Geometry: final body of the model. Coordinates: model frame, mm. Face numbers are marked on the shaded views. A direction names the side the tool comes from. Coordinates: 2 decimals unless noted, no trailing zeros. Order: outer loops, then holes, each group sorted by start corner. A loop starts at its lowest first (then second) coordinate and runs counter-clockwise, first axis right, second up. Notation, with made-up numbers: M 45.25,78 L 68.25,78 A27 ccw 68.25,98 Z; hole C 1.25,60 d9. An arc over 180 degrees is marked long. One line per question, with ' | ' between items.
Autodesk Inventor part; units mm, degrees
ref_plane "YZ Plane" through (0, 0, 0) normal (1, 0, 0) x (0, 1, 0)
ref_plane "XZ Plane" through (0, 0, 0) normal (0, 1, 0) x (-1, 0, 0)
ref_plane "XY Plane" through (0, 0, 0) normal (0, 0, 1) x (1, 0, 0)
sketch "Sketch1" plane through (0, 0, 0) normal (0, 1, 0) x (-1, 0, 0)
  line L0 (55, 40) -> (-55, 40)
  line L1 (-55, 40) -> (-55, -40)
  line L2 (-55, -40) -> (55, -40)
  line L3 (55, -40) -> (55, 40)
  line L4 (55, 40) -> (-55, -40) construction
  line L5 (-55, 40) -> (55, -40) construction
  line L6 (0, -56) -> (0, 56)
  point P0 (0, 0)
  dimension "d0" = 110
  dimension "d1" = 80
extrude "Extrusion1" add sketch "Sketch1" along normal blind 3
sketch "Sketch2" plane through (0, 3, 0) normal (0, 1, 0) x (1, 0, 0)
  line L0 (-55, 40) -> (-55, -40)
  line L1 (-55, -40) -> (55, -40)
  line L2 (55, -40) -> (55, 40)
  line L3 (49, -34) -> (-49, -34)
  line L4 (-49, -34) -> (-49, 34)
  line L5 (-49, 34) -> (49, 34)
  line L6 (49, 34) -> (49, -34)
  line L7 (49, -34) -> (-49, 34) construction
  line L8 (-49, -34) -> (49, 34) construction
  line L9 (55, 40) -> (-55, 40)
  point P0 (0, 0)
  dimension "d36" = 98
  dimension "d37" = 68
extrude "Extrusion2" add sketch "Sketch2" along normal blind 25.4125
sketch "Sketch7" plane through (-49, 3, 34) normal (1, 0, 0) x (0, 0, -1)
  circle A0 centre (31.25, 12) radius 8.25
  line L0 (74, -3) -> (-6, -3)
  circle A1 centre (31.25, 12) radius 10.25
  line L1 (21, 12) -> (41.5, 12)
  line L2 (41.5, 12) -> (41.5, 0)
  line L3 (-6, -3) -> (-6, 25.4125)
  line L4 (0, 0) -> (41.5, 0)
  line L5 (0, 0) -> (0, 25.4125)
  line L6 (21, 12) -> (21, 0)
  line L7 (68, 0) -> (0, 0)
  point P0 (34, -3)
  point P1 (54, -3)
  point P2 (0, 25.25)
  point P3 (22.1693, 16.7543)
  point P4 (23, 12)
  point P5 (39.5, 12)
  dimension "MotorDiameter" = 16.5
  dimension "d18" = 15
  dimension "d20" = 2
  dimension "d144" = 37.25
extrude "Extrusion5" add sketch "Sketch7" along normal blind 13 contours L1 A1 A0 | A0 L1 A1 | L2 L4 L6 A1
sketch "Sketch8" plane through (-36, 3, 34) normal (1, 0, 0) x (0, 0, -1)
  arc A0 (41.5, 12) -> (21, 12) centre (31.25, 12) ccw
  arc A1 (41.5, 12) -> (21, 12) centre (31.25, 12) ccw
  arc A2 (23, 12) -> (23, 12) centre (31.25, 12) ccw
  line L0 (41.5, 0) -> (21, 0)
  line L1 (21, 12) -> (21, 0)
  line L2 (41.5, 0) -> (21, 0)
  line L3 (41.5, 0) -> (41.5, 12)
  circle A3 centre (31.25, 12) radius 7.75
  line L4 (25.15, 17.5545) -> (25.15, 0)
  line L5 (31.25, 19.75) -> (31.25, 4.25)
  line L6 (37.35, 17.5545) -> (37.35, 0)
  circle A4 centre (31.25, 12) radius 8.25
  arc A5 (41.5, 12) -> (21, 12) centre (31.25, 12) ccw
  line L7 (21, 12) -> (21, 0)
  line L8 (41.5, 0) -> (21, 0)
  line L9 (41.5, 0) -> (41.5, 12)
  line L10 (37.35, 17.5545) -> (39.8645, 17.5545)
  line L11 (25.15, 17.5545) -> (22.6355, 17.5545)
  point P0 (34, -3)
  point P1 (19.75, 15)
  point P2 (37.35, 7.2196)
  point P3 (25.15, 7.2196)
  point P4 (22.6355, 17.5545)
  dimension "d145" = 15.5
  dimension "d146" = 15.5
  dimension "d147" = 12.2
extrude "Extrusion6" add sketch "Sketch8" along normal blind 20 contours L3 L0 L6 A2 L10 A0 | L11 A2 L4 L0 L1 A0 | A2 L6 A3 | L0 L4 A2 L6 | L4 A3 A2 | A3 L6 | A2 L4 A3 L6 | L4 A3 picked at (32.1563, 4.1687)
sketch "Sketch9" plane through (-49, 17, 8.75) normal (1, 0, 0) x (0, 0, -1)
  line L0 (48.75, -17) -> (-31.25, -17)
  line L1 (-31.25, -17) -> (-31.25, 11.4125)
  arc A0 (-0.1, 3.5545) -> (12.1, 3.5545) centre (6, -2) ccw
  arc A1 (12.1, 3.5545) -> (-0.1, 3.5545) centre (6, -2) ccw
  circle A2 centre (6, -2) radius 8.25
  circle A3 centre (6, -2) radius 1.75
  point P0 (8.75, -17)
  point P1 (44, -20)
  dimension "d148" = 3.5
extrude "Extrusion7" cut sketch "Sketch9" against normal up to surface (6 mm away) contours A3
mirror "Mirror2" about plane through (0, 0, 0) normal (1, 0, 0) of "Extrusion7", "Extrusion6", "Extrusion5"
sketch "Sketch28" plane through (-49, 3, -34) normal (0, 0, 1) x (1, 0, 0)
  line L0 (98, 0) -> (0, 0)
  line L1 (98, 0) -> (98, 25.4125)
  line L2 (0, 0) -> (0, 25.4125)
  line L3 (92, 19.4125) -> (92, 6)
  line L4 (92, 6) -> (6, 6)
  line L5 (6, 6) -> (6, 19.4125)
  line L6 (6, 19.4125) -> (92, 19.4125)
  circle A0 centre (6, 19.4125) radius 2
  circle A1 centre (6, 6) radius 2
  circle A2 centre (92, 19.4125) radius 2
  circle A3 centre (92, 6) radius 2
  line L7 (0, 25.4125) -> (98, 25.4125)
  point P0 (49, -3)
  dimension "d120" = 4
  dimension "d121" = 4
  dimension "d122" = 4
  dimension "d123" = 4
  dimension "d132" = 6
  dimension "d133" = 6
  dimension "d134" = 6
extrude "Extrusion24" cut sketch "Sketch28" against normal blind 2.2 contours L6 A2 L3 | L3 A2 L6 | A3 L4 L3 | L3 L4 A3 | A0 L5 L6 | L6 L5 A0 | A1 L5 L4 | L4 L5 A1
sketch "Sketch29" plane through (-43, 22.4125, -36.2) normal (0, 0, 1) x (1, 0, 0)
  circle A0 centre (0, 0) radius 2
  circle A1 centre (0, -13.4125) radius 2
  circle A2 centre (86, 0) radius 2
  circle A3 centre (86, -13.4125) radius 2
  circle A4 centre (0, 0) radius 1.1
  circle A5 centre (0, -13.4125) radius 1.1
  circle A6 centre (86, 0) radius 1.1
  circle A7 centre (86, -13.4125) radius 2
  circle A8 centre (86, -13.4125) radius 1.1
  point P0 (43, -22.4125)
  dimension "d126" = 2.2
  dimension "d127" = 2.2
  dimension "d128" = 2.2
  dimension "d129" = 2.2
extrude "Extrusion25" cut sketch "Sketch29" against normal up to surface (3.8 mm away) contours A4 | A5 | A6 | A8
sketch "Sketch30" plane through (0, 28.4125, 0) normal (0, 1, 0) x (1, 0, 0)
  line L0 (-55, 40) -> (-55, -40)
  line L1 (-55, 37) -> (54.8299, 37)
  line L2 (55, 40) -> (-55, 40)
  line L3 (-52, 40) -> (-52, -40)
  line L4 (-55, -40) -> (55, -40)
  circle A0 centre (-52, 37) radius 1.45
  line L5 (-55, -37) -> (55, -37)
  circle A1 centre (-52, -37) radius 1.45
  point P0 (0, 0)
  dimension "d135" = 3
  dimension "d136" = 3
  dimension "d137" = 2.9
  dimension "d138" = 3
  dimension "d139" = 2.9
extrude "Extrusion26" cut sketch "Sketch30" against normal blind 7 contours A0 L3 L1 | L1 L3 A0 | A0 L1 L3 | A1 L3 L5 | L5 L3 A1 | L1 A0 L3 | L5 A1 L3 | L3 A1 L5
mirror "Mirror11" about plane through (0, 0, 0) normal (1, 0, 0) of "Extrusion26"
sketch "Sketch31" plane through (49, 3, 34) normal (-1, 0, 0) x (0, 0, 1)
  line L0 (-21, 12) -> (-21, 0)
  line L1 (0, 0) -> (-21, 0)
  line L2 (0, 0) -> (0, 25.4125)
  line L3 (-68, 25.4125) -> (0, 25.4125)
  line L4 (-68, 0) -> (-68, 25.4125)
  line L5 (-41.5, 0) -> (-68, 0)
  line L6 (-41.5, 0) -> (-41.5, 12)
  arc A0 (-21, 12) -> (-41.5, 12) centre (-31.25, 12) ccw
  line L7 (-68, 25.4125) -> (0, 25.4125)
  line L8 (-65, 25.4125) -> (-65, 0)
  line L9 (-41.5, 0) -> (-68, 0)
  line L10 (-68, 0) -> (-68, 25.4125)
  circle A1 centre (-65, 18) radius 2
  circle A2 centre (-65, 6) radius 2
  point P0 (-34, -3)
  dimension "d150" = 3
  dimension "d152" = 4
  dimension "d153" = 7.4125
  dimension "d154" = 4
  dimension "d155" = 6
extrude "Extrusion27" cut sketch "Sketch31" against normal blind 2.2 contours A2 L8 | L8 A2 | A1 L8 | L8 A1
sketch "Sketch32" plane through (51.2, 21, -31) normal (-1, 0, 0) x (0, 0, 1)
  circle A0 centre (0, 0) radius 2
  circle A1 centre (0, 0) radius 2
  circle A2 centre (0, -12) radius 2
  circle A3 centre (0, -12) radius 2
  circle A4 centre (0, 0) radius 1.1
  circle A5 centre (0, -12) radius 1.1
  point P0 (31, -21)
  dimension "d158" = 2.2
  dimension "d159" = 2.2
extrude "Extrusion28" cut sketch "Sketch32" against normal up to surface (3.8 mm away) contours A4 | A5
sketch "Sketch33" plane through (49, 3, 34) normal (0, 0, -1) x (-1, 0, 0)
  line L0 (98, 0) -> (0, 0)
  line L1 (98, 0) -> (98, 25.4125)
  line L2 (0, 25.4125) -> (98, 25.4125)
  line L3 (0, 0) -> (0, 25.4125)
  line L4 (0, 25.4125) -> (98, 25.4125)
  line L5 (3, 25.4125) -> (3, 0)
  line L6 (98, 0) -> (0, 0)
  circle A0 centre (3, 18) radius 2
  circle A1 centre (3, 6) radius 2
  point P0 (49, -3)
  dimension "d162" = 3
  dimension "d163" = 4
  dimension "d164" = 4
  dimension "d165" = 7.4125
  dimension "d166" = 6
extrude "Extrusion29" cut sketch "Sketch33" against normal blind 2.2 contours A1 L5 | L5 A1 | A0 L5 | L5 A0
sketch "Sketch34" plane through (46, 21, 36.2) normal (0, 0, -1) x (-1, 0, 0)
  circle A0 centre (0, 0) radius 2
  circle A1 centre (0, -12) radius 2
  circle A2 centre (0, 0) radius 1.1
  circle A3 centre (0, -12) radius 1.1
  point P0 (46, -21)
  dimension "d169" = 2.2
  dimension "d170" = 2.2
extrude "Extrusion30" cut sketch "Sketch34" against normal up to surface (3.8 mm away) contours A2 | A3
mirror "Mirror13" about plane through (0, 0, 0) normal (1, 0, 0) of "Extrusion27", "Extrusion28", "Extrusion29", "Extrusion30"
equation "\"d0\" = BoxWidth"
equation "\"d1\" = BoxLength"
equation "\"d2\" = BaseThickness"
equation "\"d37\" = BoxLength - 2 * SideThickness"
equation "\"d18\" = DriveMotorHeight"
equation "\"d20\" = DriveMotorMountThickness"
equation "\"SideThickness\" = 6"
equation "\"BaseThickness\" = 3"
equation "\"TopThickness\" = 1.5875"
equation "\"BoxWidth\" = 110"
equation "\"BoxLength\" = 80"
equation "\"Height\" = 30"
equation "\"DriveMotorHeight\" = 0.5 * Height"
equation "\"DriveMotorMountThickness\" = 2"
equation "\"ScrewDia\" = 2.9"
equation "\"ScrewDepth\" = 7"
equation "\"ForkScrewHeadDia\" = 4"
equation "\"ForkScrewDia\" = 2.2"
equation "\"ForkScrewHeadDepth\" = 2.2"
equation "\"DriveMotorOffset\" = 37.25"
equation "\"DriveMotorDia\" = 16.5"
equation "\"SideArmorWidth\" = 15"
equation "\"ForkLength\" = 60"
equation "\"WheelWidth\" = 16.51"
equation "\"DriveMotorHoleDia\" = 3.5"
equation "\"ForkPlugDia\" = 3.5"
equation "\"ForkPlugTolerance\" = 0.5"
equation "\"ForkPlugLength\" = 3"
properties part number "BodyWedgeBaseV3.1" material "Thermoplastic Resin"
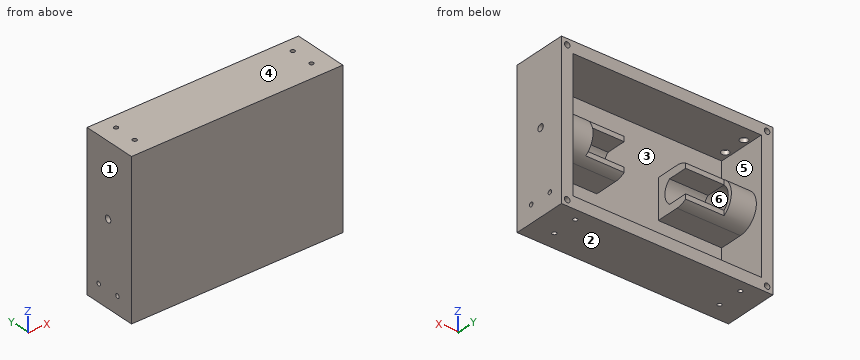
1. Draft query along X for the marked faces 1, 2 and 3. Return one class per face: pulls with the +X half, pulls with the -X half, needs draft (parallel to the pull), parting line crosses it, or undercut.
Response values:
face 1: pulls with the -X half | face 2: needs draft | face 3: undercut
2. Section C-C, the plane x = 31.5. Output: boundary loops of the cut face in (y, z).
Response values:
outline: M 0,-40 L 28.41,-40 L 28.41,-34 L 3,-34 L 3,-7.5 L 15,-7.5 A10.25 ccw 20.55,-5.86 L 20.55,-3.35 L 10.22,-3.35 A7.75 cw 10.22,8.85 L 20.55,8.85 L 20.55,11.36 A10.25 ccw 15,13 L 3,13 L 3,34 L 28.41,34 L 28.41,40 L 0,40 Z
3. Access query for the marked faces 4, 5 and 6. Directions: +Z, -Z, +X, -X, +Y, -Y. A direction counts if a zero-diameter tool reaches every point of the face in a straight line with its end or side. Return the directions, or none.
Response values:
face 4: +Z, +X, -X, +Y, -Y | face 5: +Y | face 6: none
4. Material intervals for line 1 (Z direction, x = -40, y = 3.25); line 2 (Z direction, x = 30.5, y = 13); line 3 (Y direction, x = 50.45, z = -31), sorted ascending. Write a range as [from, to].
Response values:
line 1: z = [-40, -34], [-7.5, 13], [34, 40] | line 2: z = [-40, -34], [-7.5, -3.35], [8.85, 13], [34, 40] | line 3: y = [0, 7], [11, 19], [23, 28.41]
5. Section A-A, the plane x = 12. Output: boundary loops of the cut face in (y, z).
Response values:
outline: M 0,-40 L 28.41,-40 L 28.41,-34 L 3,-34 L 3,34 L 28.41,34 L 28.41,40 L 0,40 Z
6. Section D-D, the plane z = 6.5. Output: boundary loops of the cut face in (x, y), and give its area (3 significant figures).
Response values:
outline: M -55,0 L 55,0 L 55,28.41 L 49,28.41 L 49,24.54 L 36,24.54 L 36,22.35 L 49,22.35 L 49,7.65 L 36,7.65 L 36,8.22 L 16,8.22 L 16,3 L -16,3 L -16,8.22 L -36,8.22 L -36,7.65 L -49,7.65 L -49,22.35 L -36,22.35 L -36,24.54 L -49,24.54 L -49,28.41 L -55,28.41 Z | area: 1,020 mm^2
7. Pin query (flat end, axial travel): P1, Ø1.5, axis at x = 35, z = -31.5, coming from the +Y side. Return the tip coordinate at first contact, or that it passes through.
Response values:
P1: stops at y = 3
8. Section B-B, the plane z = -25.5. Output: boundary loops of the cut face in (x, y), and give its area (3 significant figures).
Response values:
outline: M -55,0 L 55,0 L 55,28.41 L 49,28.41 L 49,3 L -49,3 L -49,28.41 L -55,28.41 Z | area: 635 mm^2
